Geometry check sheet. Reference: drawing and pictorial views, mm from the part's lowest x, y, z. Give positions to 0.01 mm unless a question says otherwise; leave off trailing zeros. Write each loop counter-clockwise with the first axis right and the second up, starting at its lowest first coordinate (ties: lowest second). Pieces come first, ordered by that corner, then holes. Notation, with made-up numbers: (-26, 13) - (30, 13) arc R15 ccw to (30, 27) - close; hole circle Ø9 at (62.25, -11.75). An arc over 180 degrees is marked (long way). Put each result on its own line as item: value.
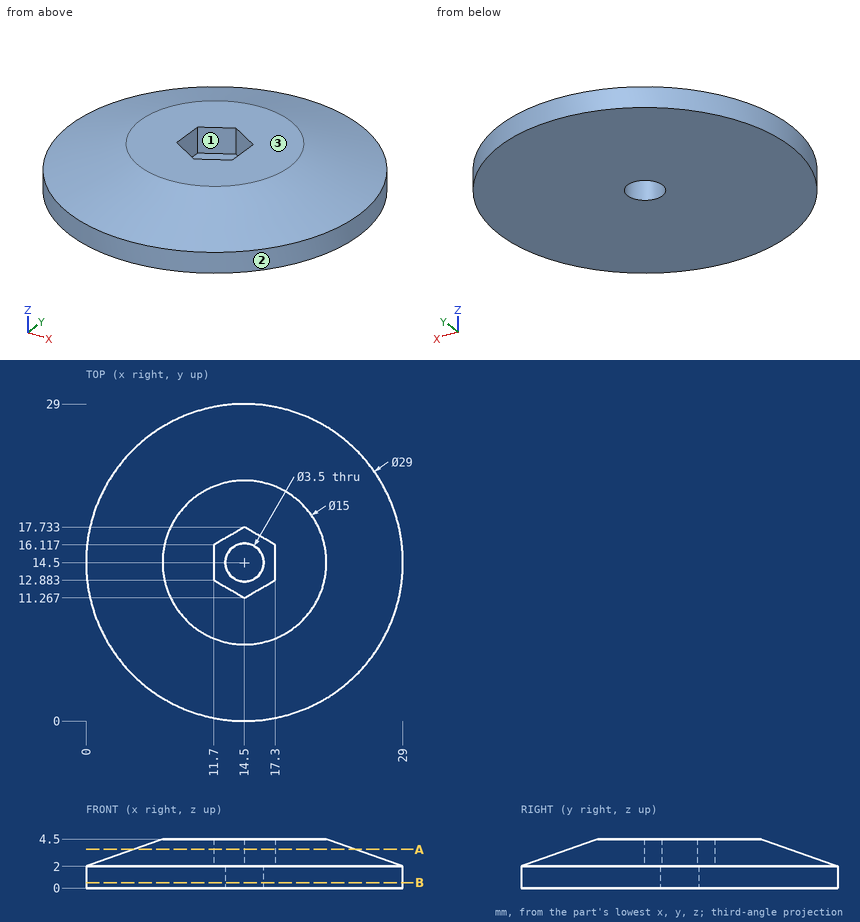
Q1. Section check A-A, the plane z = 3.55. Record the cut outline in (x, y), plus the area to 3 significant figures.
Answers follow:
outline: circle Ø20.32 at (14.5, 14.5); hole (11.7, 12.88) - (14.5, 11.27) - (17.3, 12.88) - (17.3, 16.12) - (14.5, 17.73) - (11.7, 16.12) - close
area: 297 mm2
Q2. Section check B-B, the plane z = 0.5. Record the cut outline in (x, y), plus the area to 3 significant figures.
Answers follow:
outline: circle Ø29 at (14.5, 14.5); hole circle Ø3.5 at (14.5, 14.5)
area: 651 mm2
Q3. Go/stop test with flat-tipped pins: pin 1 Ø1.5 at (y, z) = (11, 1) entering from -X; pin 2 Ø2 at (x, z) = (5, 2) entering from +Y; pin 3 Ø1 at (y, z) = (24.5, 2) entering from +X (1 decimal). Record where each tip stops, or that it passes through.
Answers follow:
pin 1: stops at x = 0.26
pin 2: stops at y = 26.25
pin 3: stops at x = 25.5
Q4. Release check for a two-part mould opening along X. For the marked faces 1, 2 and 3 record: released by +X, released by -X, zero draft, split by the parting line, or undercut.
Answers follow:
face 1: undercut
face 2: split by the parting line
face 3: zero draft
Q5. Scan lines: line 1 along Y through (x, z) = (14.5, 1); line 2 along Z through (x, y) = (15.75, 16.5); line 3 along Y through (x, z) = (22.25, 1.1) (1 decimal). Record each from-to range of solid material in increasing order.
Answers follow:
line 1: y = 0 to 12.75, 16.25 to 29
line 2: z = 0 to 2
line 3: y = 2.2 to 26.8
